Source: CAD feature listing. Evaluate the final solid. Frame: model axes, mm. A direction names the side the tool comes from. Give positions to 0.01 mm unless a question says otherwise; leave off trailing zeros. Order: outer loops, then holes, each group sorted by start corner. A loop starts at its lowest first (then second) coordinate and runs counter-clockwise, first axis right, second up.
from build123d import *

# Parameters (mm, degrees)
SKETCH_1_W          = 15
SKETCH_1_H          = 15
SKETCH_1_W_2        = 13
SKETCH_1_H_2        = 13
EXTRUDE_1_DEPTH     = 570
SKETCH_2_R          = 1.45
CUT_EXTRUDE_1_DEPTH = 571.246657158
SKETCH_3_R          = 1.45
CUT_EXTRUDE_2_DEPTH = 571.246657158


with BuildPart() as part:
    # 草图1 → 凸台-拉伸1 (new body)
    with BuildSketch(Plane(origin=(0, 0, 0), x_dir=(0, 0, -1), z_dir=(1, 0, 0))):
        Rectangle(SKETCH_1_W, SKETCH_1_H)
        Rectangle(SKETCH_1_W_2, SKETCH_1_H_2, mode=Mode.SUBTRACT)
    extrude(amount=EXTRUDE_1_DEPTH)

    # 草图2 → 切除-拉伸1 (cut, through all)
    with BuildSketch(Plane(origin=(0, 7.5, 0), x_dir=(1, 0, 0), z_dir=(0, 1, 0))):
        with Locations(Location((20, 0, 0), (0, 0, 270))):
            Circle(SKETCH_2_R)
        with Locations(Location((40, 0, 0), (0, 0, 270))):
            Circle(SKETCH_2_R)
        with Locations(Location((60, 0, 0), (0, 0, 270))):
            Circle(SKETCH_2_R)
        with Locations(Location((80, 0, 0), (0, 0, 270))):
            Circle(SKETCH_2_R)
        with Locations(Location((100, 0, 0), (0, 0, 270))):
            Circle(SKETCH_2_R)
        with Locations(Location((120, 0, 0), (0, 0, 270))):
            Circle(SKETCH_2_R)
        with Locations(Location((140, 0, 0), (0, 0, 270))):
            Circle(SKETCH_2_R)
        with Locations(Location((160, 0, 0), (0, 0, 270))):
            Circle(SKETCH_2_R)
        with Locations(Location((180, 0, 0), (0, 0, 270))):
            Circle(SKETCH_2_R)
        with Locations(Location((200, 0, 0), (0, 0, 270))):
            Circle(SKETCH_2_R)
        with Locations(Location((220, 0, 0), (0, 0, 270))):
            Circle(SKETCH_2_R)
        with Locations(Location((240, 0, 0), (0, 0, 270))):
            Circle(SKETCH_2_R)
        with Locations(Location((260, 0, 0), (0, 0, 270))):
            Circle(SKETCH_2_R)
        with Locations(Location((280, 0, 0), (0, 0, 270))):
            Circle(SKETCH_2_R)
        with Locations(Location((300, 0, 0), (0, 0, 270))):
            Circle(SKETCH_2_R)
        with Locations(Location((320, 0, 0), (0, 0, 270))):
            Circle(SKETCH_2_R)
        with Locations(Location((340, 0, 0), (0, 0, 270))):
            Circle(SKETCH_2_R)
        with Locations(Location((360, 0, 0), (0, 0, 270))):
            Circle(SKETCH_2_R)
        with Locations(Location((380, 0, 0), (0, 0, 270))):
            Circle(SKETCH_2_R)
        with Locations(Location((400, 0, 0), (0, 0, 270))):
            Circle(SKETCH_2_R)
        with Locations(Location((420, 0, 0), (0, 0, 270))):
            Circle(SKETCH_2_R)
        with Locations(Location((440, 0, 0), (0, 0, 270))):
            Circle(SKETCH_2_R)
        with Locations(Location((460, 0, 0), (0, 0, 270))):
            Circle(SKETCH_2_R)
        with Locations(Location((480, 0, 0), (0, 0, 270))):
            Circle(SKETCH_2_R)
        with Locations(Location((500, 0, 0), (0, 0, 270))):
            Circle(SKETCH_2_R)
        with Locations(Location((520, 0, 0), (0, 0, 270))):
            Circle(SKETCH_2_R)
        with Locations(Location((540, 0, 0), (0, 0, 270))):
            Circle(SKETCH_2_R)
        with Locations(Location((560, 0, 0), (0, 0, 270))):
            Circle(SKETCH_2_R)
    extrude(amount=-CUT_EXTRUDE_1_DEPTH, mode=Mode.SUBTRACT)

    # 草图3 → 切除-拉伸2 (cut, through all)
    with BuildSketch(Plane.XY.offset(7.5)):
        with Locations((5, 0)):
            Circle(SKETCH_3_R)
        with Locations((15, 0)):
            Circle(SKETCH_3_R)
        with Locations((565, 0)):
            Circle(SKETCH_3_R)
        with Locations((555, 0)):
            Circle(SKETCH_3_R)
        with Locations((30, 0)):
            Circle(SKETCH_3_R)
        with Locations((50, 0)):
            Circle(SKETCH_3_R)
        with Locations((70, 0)):
            Circle(SKETCH_3_R)
        with Locations((90, 0)):
            Circle(SKETCH_3_R)
        with Locations((110, 0)):
            Circle(SKETCH_3_R)
        with Locations((130, 0)):
            Circle(SKETCH_3_R)
        with Locations((150, 0)):
            Circle(SKETCH_3_R)
        with Locations((170, 0)):
            Circle(SKETCH_3_R)
        with Locations((190, 0)):
            Circle(SKETCH_3_R)
        with Locations((210, 0)):
            Circle(SKETCH_3_R)
        with Locations((230, 0)):
            Circle(SKETCH_3_R)
        with Locations((250, 0)):
            Circle(SKETCH_3_R)
        with Locations((270, 0)):
            Circle(SKETCH_3_R)
        with Locations((290, 0)):
            Circle(SKETCH_3_R)
        with Locations((310, 0)):
            Circle(SKETCH_3_R)
        with Locations((330, 0)):
            Circle(SKETCH_3_R)
        with Locations((350, 0)):
            Circle(SKETCH_3_R)
        with Locations((370, 0)):
            Circle(SKETCH_3_R)
        with Locations((390, 0)):
            Circle(SKETCH_3_R)
        with Locations((410, 0)):
            Circle(SKETCH_3_R)
        with Locations((430, 0)):
            Circle(SKETCH_3_R)
        with Locations((450, 0)):
            Circle(SKETCH_3_R)
        with Locations((470, 0)):
            Circle(SKETCH_3_R)
        with Locations((490, 0)):
            Circle(SKETCH_3_R)
        with Locations((510, 0)):
            Circle(SKETCH_3_R)
        with Locations((530, 0)):
            Circle(SKETCH_3_R)
    extrude(amount=-CUT_EXTRUDE_2_DEPTH, mode=Mode.SUBTRACT)


solid = part.part
(1) Access query for faces 1 (the flat face through (281, 0, -7.5)), 2 (the flat face through (281, -6.5, 2)). Directions: +Z, -Z, +X, -X, +Y, -Y. A direction counts if a zero-diameter tool reaches every point of the face in a straight line with its end or side. Return the directions, or none.
(2) Draft query along Y for faces 3 (the flat face through (281, 7.5, 2)), 4 (the flat face through (281, 0, 7.5)), 5 (the flat face through (281, 6.5, 2)), 6 (the flat face through (281, -7.5, 2)). Return one class per face: +Y half, -Y half, draft (parallel to the pull), parting line (faces both ways), or undercut.
(3) Line query: line 1 along Z through (x, y) = (274, -1.75); line 2 along Z through (x, y) = (380, 7.2). Output: solid intervals per line, ascending.
(4) Section A-A, the plane z = 3.75. Return loops of the section in (x, y).
(5) Pin query (flat end, axial travel): pin 1 Ø4.5 at (x, z) = (440, 0) entering from +Y; pin 2 Ø2.5 at (x, y) = (130, 0) entering from -Z. Return the tip coordinate at first contact, or that it passes through.
Checks:
1. face 1: -Z, +X, -X, +Y, -Y
1. face 2: +X, -X
2. face 3: +Y half
2. face 4: draft
2. face 5: undercut
2. face 6: -Y half
3. line 1: z = -7.5 to -6.5, 6.5 to 7.5
3. line 2: z = -7.5 to -1.45, 1.45 to 7.5
4. outline: (0, -7.5) - (570, -7.5) - (570, -6.5) - (0, -6.5) - close; (0, 6.5) - (570, 6.5) - (570, 7.5) - (0, 7.5) - close
5. pin 1: stops at y = 7.5
5. pin 2: passes through
